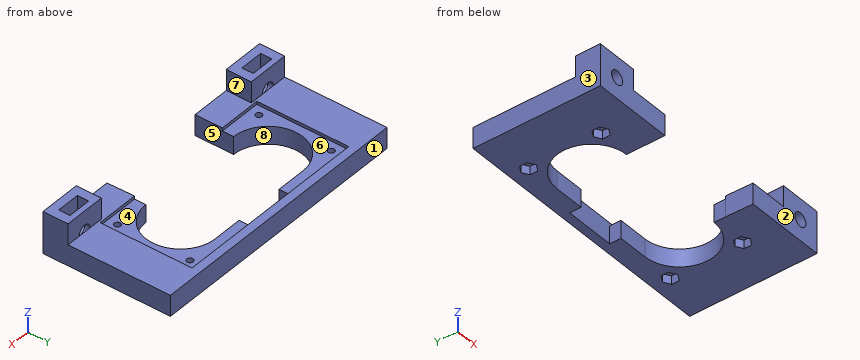
```python
from build123d import *

# Parameters (mm, degrees)
EXTRUDE_1_DEPTH      = 5
SKETCH_1_R           = 0.75
CUT_EXTRUDE_11_DEPTH = 5
SKETCH_3_W           = 47
SKETCH_3_H           = 22
CUT_EXTRUDE_14_DEPTH = 0.73
SKETCH_4_W           = 10
SKETCH_4_H           = 10
EXTRUDE_2_DEPTH      = 6
SKETCH_5_R           = 1.65
CUT_EXTRUDE_15_DEPTH = 6
CUT_EXTRUDE_16_DEPTH = 2.7
CUT_EXTRUDE_17_DEPTH = 2


with BuildPart() as part:
    # Эскиз2 → Бобышка-Вытянуть1 (new body)
    with BuildSketch(Plane.XY):
        Polygon((-32.499999999, 13), (32.500000001, 13), (32.500000001, -17.5), (13.323102298, -17.5), (13.16, -11), (-13.16, -11), (-13.16, -17.5), (-32.499999999, -17.5), align=None)
    extrude(amount=EXTRUDE_1_DEPTH)

    # Эскиз1 → Вырез-Вытянуть11 (cut)
    with BuildSketch(Plane.XY):
        with Locations((21.22, 8.675)):
            Circle(SKETCH_1_R)
        with Locations(Location((21.22, -8.675, 0), (0, 0, 180))):
            Circle(SKETCH_1_R)
        with Locations((-21.22, -8.675)):
            Circle(SKETCH_1_R)
        with Locations(Location((-21.22, 8.675, 0), (0, 0, 180))):
            Circle(SKETCH_1_R)
        with BuildLine():
            Line((13.16, 8.3), (6, 8.3))
            Line((6, 8.3), (6, 11))
            Line((6, 11), (-6, 11))
            Line((-6, 11), (-6, 8.3))
            Line((-6, 8.3), (-13.16, 8.3))
            ThreePointArc((-13.16, 8.3), (-21.46, 0), (-13.16, -8.3))
            Line((-13.16, -8.3), (-13.16, -11))
            Line((-13.16, -11), (13.16, -11))
            Line((13.16, -11), (13.16, -8.3))
            ThreePointArc((13.16, -8.3), (21.46, 0), (13.16, 8.3))
        make_face()
    extrude(amount=CUT_EXTRUDE_11_DEPTH, mode=Mode.SUBTRACT)

    # Эскиз3 → Вырез-Вытянуть14 (cut)
    with BuildSketch(Plane.XY.offset(5)):
        Rectangle(SKETCH_3_W, SKETCH_3_H)
    extrude(amount=-CUT_EXTRUDE_14_DEPTH, mode=Mode.SUBTRACT)

    # Эскиз4 → Бобышка-Вытянуть2 (add)
    with BuildSketch(Plane.XZ.offset(17.5)):
        with Locations((-27.499999999, 5)):
            Rectangle(SKETCH_4_W, SKETCH_4_H)
        with Locations((27.500000001, 5)):
            Rectangle(SKETCH_4_W, SKETCH_4_H)
    extrude(amount=-EXTRUDE_2_DEPTH)

    # Эскиз5 → Вырез-Вытянуть15 (cut)
    with BuildSketch(Plane.XZ.offset(17.5)):
        with Locations((-27.499999999, 5)):
            Circle(SKETCH_5_R)
        with Locations((27.500000001, 5)):
            Circle(SKETCH_5_R)
    extrude(amount=-CUT_EXTRUDE_15_DEPTH, mode=Mode.SUBTRACT)

    # Эскиз6 → Вырез-Вытянуть16 (cut)
    with BuildSketch(Plane(origin=(0, -15.5, 0), x_dir=(-1, 0, 0), z_dir=(0, -1, 0))):
        Polygon((30.299999999, -6.616580754), (30.299999999, -10), (24.699999999, -10), (24.699999999, -6.616580754), (24.699999999, -3.383419246), (27.499999999, -1.766838493), (30.299999999, -3.383419246), align=None)
        Polygon((-24.700000001, -6.616580754), (-24.700000001, -10), (-30.300000001, -10), (-30.300000001, -6.616580754), (-30.300000001, -3.383419246), (-27.500000001, -1.766838493), (-24.700000001, -3.383419246), align=None)
    extrude(amount=-CUT_EXTRUDE_16_DEPTH, mode=Mode.SUBTRACT)

    # Эскиз7 → Вырез-Вытянуть17 (cut)
    with BuildSketch(Plane(origin=(0, 0, 0), x_dir=(-1, 0, 0), z_dir=(0, 0, -1))):
        Polygon((-21.22, 10.522520861), (-22.82, 9.598760431), (-22.82, 7.751239569), (-21.22, 6.827479139), (-19.62, 7.751239569), (-19.62, 9.598760431), align=None)
        Polygon((-21.22, -6.827479139), (-22.82, -7.751239569), (-22.82, -9.598760431), (-21.22, -10.522520861), (-19.62, -9.598760431), (-19.62, -7.751239569), align=None)
        Polygon((21.22, 10.522520861), (19.62, 9.598760431), (19.62, 7.751239569), (21.22, 6.827479139), (22.82, 7.751239569), (22.82, 9.598760431), align=None)
        Polygon((21.22, -6.827479139), (19.62, -7.751239569), (19.62, -9.598760431), (21.22, -10.522520861), (22.82, -9.598760431), (22.82, -7.751239569), align=None)
    extrude(amount=-CUT_EXTRUDE_17_DEPTH, mode=Mode.SUBTRACT)


solid = part.part
```
The listing builds one solid part. Answer for the finished solid, in the listing's coordinates (mm). Face numbers are marked on the shaded views. A direction names the side the tool comes from. Give positions to 0.01 mm unless a question says otherwise; leave off trailing zeros. Order: outer loops, then holes, each group sorted by start corner. A loop starts at its lowest first (then second) coordinate and runs counter-clockwise, first axis right, second up. Notation, with made-up numbers: (-23.75, -8) -> (31.25, -8) arc R33 cw to (31.25, 29) -> close; hole circle Ø6 at (5.5, 53.25). An arc over 180 degrees is marked (long way). Answer as a JSON object with one key per item and string values. Group by question number.
Item 1: A tool of negligible diameter and unlimited length cuts with its end or side. For the marked faces 5, 6, 7 and 8, from which of +Z, -Z, +X, -X, +Y, -Y can it reach the whole face along a straight path? Write none if from no direction.
Item 2: Flat-ended cylindrical pins translate along their axes: pin 1 (1.3 mm diameter, centred on x = -11, z = 2, fed in from -Y); pin 2 (9 mm diameter, centred on x = 18, y = -4.5, fed in from +Z); pin 3 (14 mm diameter, centred on x = -15, y = 5, fed in from +Z). Find the tip coordinate at first contact, or state that the pin passes through.
Item 3: The part is cut by section D-D on z = 2.75. Write down the section's boundary in (x, y) (3 decimals).
Item 4: The part is cut by section A-A on z = 8.5. Write down the section's boundary in (x, y), and give its area (3 significant figures).
Item 5: Consider L1, parallel to Z at x = 27.5, y = -16.05; L2, parallel to X at y = 7.5, z = 4.75; L3, parallel to X at y = -14, z = 4. Determine where each line is inside the solid, lowest interval first. Write a range as from..to.
Item 6: The part is cut by section C-C on x = -10. Write down the section's boundary in (y, z), and give its area (3 significant figures).
Item 7: The part is cut by section B-B on y = 0. Write down the section's boundary in (x, z).
Item 8: Determine the mould class of the marked faces 1, 2, 3 and 4 for opening direction Y: pulls with the +Y half, pulls with the -Y half, needs draft (parallel to the pull), parting line crosses it, or undercut.
Result set:
{
 "1": {"face 5": "+Z, -Z, -Y", "face 6": "+Z", "face 7": "+Z, +Y, -Y", "face 8": "+Z, -Z"},
 "2": {"pin 1": "y = 8.3", "pin 2": "z = 4.27", "pin 3": "z = 5"},
 "3": {"outline": "(-32.5, -17.5) -> (-13.16, -17.5) -> (-13.16, -8.3) arc R8.3 cw to (-13.16, 8.3) -> (-6, 8.3) -> (-6, 11) -> (6, 11) -> (6, 8.3) -> (13.16, 8.3) arc R8.3 cw to (13.16, -8.3) -> (13.16, -11) -> (13.323, -17.5) -> (32.5, -17.5) -> (32.5, 13) -> (-32.5, 13) -> close; hole (-29.203, -15.5) -> (-25.797, -15.5) -> (-25.797, -12.8) -> (-29.203, -12.8) -> close; hole circle Ø1.5 at (-21.22, -8.675); hole circle Ø1.5 at (-21.22, 8.675); hole circle Ø1.5 at (21.22, -8.675); hole circle Ø1.5 at (21.22, 8.675); hole (25.797, -15.5) -> (29.203, -15.5) -> (29.203, -12.8) -> (25.797, -12.8) -> close"},
 "4": {"outline": "(-32.5, -17.5) -> (-22.5, -17.5) -> (-22.5, -11.5) -> (-32.5, -11.5) -> close; (22.5, -17.5) -> (32.5, -17.5) -> (32.5, -11.5) -> (22.5, -11.5) -> close; hole (-30.3, -15.5) -> (-24.7, -15.5) -> (-24.7, -12.8) -> (-30.3, -12.8) -> close; hole (24.7, -15.5) -> (30.3, -15.5) -> (30.3, -12.8) -> (24.7, -12.8) -> close", "area": "89.8 mm²"},
 "5": {"L1": "0..3.35, 6.65..10", "L2": "-32.5..-23.5, 23.5..32.5", "L3": "-32.5..-30.3, -24.7..-13.16, 13.24..24.7, 30.3..32.5"},
 "6": {"outline": "(8.3, 0) -> (13, 0) -> (13, 5) -> (11, 5) -> (11, 4.27) -> (8.3, 4.27) -> close", "area": "21.5 mm²"},
 "7": {"outline": "(-32.5, 0) -> (-21.46, 0) -> (-21.46, 4.27) -> (-23.5, 4.27) -> (-23.5, 5) -> (-32.5, 5) -> close; (21.46, 0) -> (32.5, 0) -> (32.5, 5) -> (23.5, 5) -> (23.5, 4.27) -> (21.46, 4.27) -> close"},
 "8": {"face 1": "pulls with the +Y half", "face 2": "pulls with the -Y half", "face 3": "needs draft", "face 4": "undercut"}
}
